Work out the finished part from the listing and answer in its coordinate system (mm). Face numbers are marked on the shaded views. A direction names the side the tool comes from. Coordinates: 2 decimals unless noted, no trailing zeros. Write each loop counter-clockwise with the first axis right and the second up, starting at its lowest first coordinate (ties: lowest second). Pieces come first, ordered by that corner, then holes. Notation, with made-up numbers: (54.25, 29.5) - (98.25, 29.5) arc R34 cw to (98.25, 66.5) - close; hole circle Ø6 at (85.5, 61.25). An arc over 180 degrees is marked (long way). Answer as a JSON object with one key per item and string values. Group by question number.
from build123d import *

# Parameters (mm, degrees)
F0_R     = 15.5
F0_R_2   = 12.5
F1_DEPTH = 7.5
F2_R     = 26
F2_R_2   = 22.5
F3_DEPTH = 7.5
F4_R     = 5
F5_DEPTH = 5.5


with BuildPart() as f1:
    # F0 (on Front) → F1 (new body, symmetric)
    with BuildSketch(Plane.XZ):
        Circle(F0_R)
        Circle(F0_R_2, mode=Mode.SUBTRACT)
    extrude(amount=F1_DEPTH, both=True)



with BuildPart() as f3:
    # F2 (on Front) → F3 (new body, symmetric)
    with BuildSketch(Plane.XZ):
        Circle(F2_R)
        Circle(F2_R_2, mode=Mode.SUBTRACT)
    extrude(amount=F3_DEPTH, both=True)


with BuildPart() as f1_1:
    add(f1.part)

    add(f3.part)  # F5 merges F3
    # F4 (on Front) → F5 (join, symmetric)
    with BuildSketch(Plane.XZ):
        with Locations((-13.4350288425, 13.4350288425)):
            Circle(F4_R)
        with Locations((0, 19)):
            Circle(F4_R)
        with Locations((13.4350288425, 13.4350288425)):
            Circle(F4_R)
        with Locations((19, 0)):
            Circle(F4_R)
        with Locations((-19, 0)):
            Circle(F4_R)
        with Locations((-13.4350288425, -13.4350288425)):
            Circle(F4_R)
        with Locations((13.4350288425, -13.4350288425)):
            Circle(F4_R)
        with Locations((0, -19)):
            Circle(F4_R)
    extrude(amount=F5_DEPTH, both=True)


solid = f1_1.part
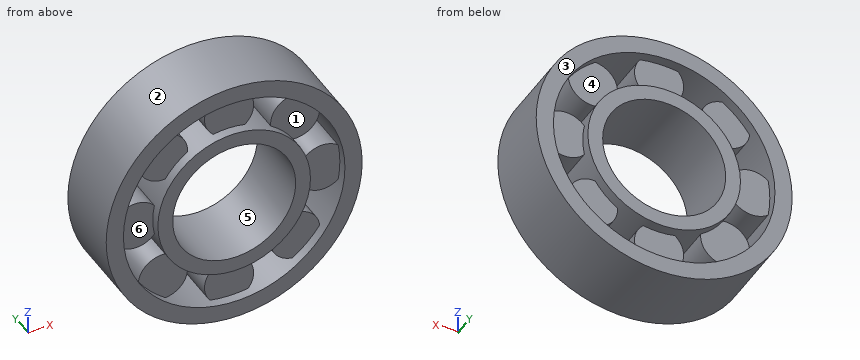
Q1. Flat-ended cylindrical pins translate along their axes: pin 1 Ø3 at (x, y) = (16, -4.5) entering from +Z; pin 2 Ø1.5 at (x, y) = (-15.5, -5) entering from -Z; pin 3 Ø3 at (x, z) = (-13, -14.5) entering from +Y; pin 4 Ø22.5 at (x, z) = (0, 0) entering from -Y. Find the tip coordinate at first contact, or state that the pin passes through.
Q2. Section C-C on x = -17 is taken. Determine the outline of the cut face in (y, z), plus the area to 3 significant figures.
Q3. Section A-A on z = 0 is taken. Determine the outline of the cut face in (x, y).
Q4. Section D-D on z = -14 is taken. Determine the outline of the cut face in (x, y), plus the area to 3 significant figures.
Q5. Consider L1, parallel to Z at x = 0, y = -2.25; L2, parallel to Z at x = -20, y = 0.5; L3, parallel to Z at x = 19, y = 0. Determine where each line is inside the solid, lowest interval first. Write a range as from..to.
Q6. Section B-B on x = 0 is taken. Determine the outline of the cut face in (y, z), plus the area to 3 significant figures.
Q7. A tool of negligible diameter and unlimited length cuts with its end or side. For the marked faces 4, 5 and 6, from which of +Z, -Z, +X, -X, +Y, -Y can it reach the whole face along a straight path? Write none if from no direction.
Q8. For a pull along Z with two mould halves and no side action, classify the marked faces 1, 2 and 3 as +Z half, -Z half, draft (parallel to the pull), parting line (faces both ways), or undercut.
Numbers:
{
 "1": {"pin 1": "stops at z = 21.58", "pin 2": "stops at z = -21.41", "pin 3": "stops at y = 5.5", "pin 4": "passes through"},
 "2": {"outline": "(-7.5, -19.67) - (7.5, -19.67) - (7.5, -14.74) - (5.5, -14.74) - (5.5, -9.93) - (-5.5, -9.93) - (-5.5, -14.74) - (-7.5, -14.74) - close; (-7.5, 14.74) - (-5.5, 14.74) - (-5.5, 9.93) - (5.5, 9.93) - (5.5, 14.74) - (7.5, 14.74) - (7.5, 19.67) - (-7.5, 19.67) - close; (-5.5, -4.58) - (5.5, -4.58) - (5.5, 4.58) - (-5.5, 4.58) - close", "area": "355 mm²"},
 "3": {"outline": "(-26, -7.5) - (-22.5, -7.5) - (-22.5, -5.5) - (-15.5, -5.5) - (-15.5, -7.5) - (-12.5, -7.5) - (-12.5, 7.5) - (-15.5, 7.5) - (-15.5, 5.5) - (-22.5, 5.5) - (-22.5, 7.5) - (-26, 7.5) - close; (12.5, -7.5) - (15.5, -7.5) - (15.5, -5.5) - (22.5, -5.5) - (22.5, -7.5) - (26, -7.5) - (26, 7.5) - (22.5, 7.5) - (22.5, 5.5) - (15.5, 5.5) - (15.5, 7.5) - (12.5, 7.5) - close"},
 "4": {"outline": "(-21.91, -7.5) - (-17.61, -7.5) - (-17.61, -5.5) - (-8.47, -5.5) - (-8.47, 5.5) - (-17.61, 5.5) - (-17.61, 7.5) - (-21.91, 7.5) - close; (-6.65, -7.5) - (6.65, -7.5) - (6.65, 7.5) - (-6.65, 7.5) - close; (8.47, -5.5) - (17.61, -5.5) - (17.61, -7.5) - (21.91, -7.5) - (21.91, 7.5) - (17.61, 7.5) - (17.61, 5.5) - (8.47, 5.5) - close", "area": "530 mm²"},
 "5": {"L1": "z = -26..-12.5, 12.5..26", "L2": "z = -16.61..-10.31, -4.9..4.9, 10.31..16.61", "L3": "z = -17.75..-12.05, -5..5, 12.05..17.75"},
 "6": {"outline": "(-7.5, -26) - (7.5, -26) - (7.5, -22.5) - (5.5, -22.5) - (5.5, -15.5) - (7.5, -15.5) - (7.5, -12.5) - (-7.5, -12.5) - (-7.5, -15.5) - (-5.5, -15.5) - (-5.5, -22.5) - (-7.5, -22.5) - close; (-7.5, 12.5) - (7.5, 12.5) - (7.5, 15.5) - (5.5, 15.5) - (5.5, 22.5) - (7.5, 22.5) - (7.5, 26) - (-7.5, 26) - (-7.5, 22.5) - (-5.5, 22.5) - (-5.5, 15.5) - (-7.5, 15.5) - close", "area": "349 mm²"},
 "7": {"face 4": "+Y", "face 5": "+Y, -Y", "face 6": "-Y"},
 "8": {"face 1": "undercut", "face 2": "parting line", "face 3": "draft"}
}
